The listing builds one solid part. Answer for the finished solid, in the listing's coordinates (mm). A direction names the side the tool comes from. Give positions to 0.01 mm unless a question says otherwise; leave off trailing zeros. One line per question, with ' | ' between items. Start each with the question number.
1. A cutting plane is placed at A-A (z = 21.5). State how many separate pieces and enclosed holes the cut face has, then the cut area to 3 significant figures.
2. Given P1, Ø4.5, axis at x = -23.89, y = 1.91, coming from the +Z side; P2, Ø0.8, axis at x = -17.5, z = 77, coming from the +Y side, each flat-ended and moving along its own axis, determine where each tip first touches the part or whether it passes through.
3. Find the intervals of material crossed by L1, parallel to X at y = 2, z = 43.5; L2, parallel to X at y = 3.75, z = 32; L3, parallel to X at y = 0, z = 39, in increasing order. Write a range as from..to.
4. For faces 1 (the face through (1, 2, 0)), 2 (the face through (-28.891, 4, 60)), determine the directions among +Z, -Z, +X, -X, +Y, -Y from which every point of the face is accessible in a straight line to the end or side of a thin tool.
5. The mould has two halves that part along X. Classify faces 3 (the face through (-18.891, 4, 60)), 4 (the face through (36.109, 2, 60)), 5 (the face through (1, -3.09, 60)): +X half, -X half, draft (parallel to the pull), parting line (faces both ways), or undercut.
```python
from build123d import *

# Parameters (mm, degrees)
ESQUISSE1_R        = 2.8
BOSS_EXTRU_1_DEPTH = 122
CONG_1_R           = 1
CONG_2_R           = 2


with BuildPart() as part:
    # Esquisse1 → Boss.-Extru.1 (new body)
    with BuildSketch(Plane.XY):
        Polygon((-35.89112663, -3.089603204), (-35.89112663, 6.910396796), (-31.89112663, 6.910396796), (-31.89112663, 0.910396796), (-28.89112663, 0.910396796), (-28.89112663, 6.910396796), (-18.89112663, 6.910396796), (-18.89112663, 0.910396796), (-15.89112663, 0.910396796), (-15.89112663, 6.910396796), (23.10887337, 6.910396796), (23.10887337, 0.910396796), (26.10887337, 0.910396796), (26.10887337, 6.910396796), (36.10887337, 6.910396796), (36.10887337, -3.089603204), align=None)
        with Locations((-23.89112663, 1.910396796)):
            Circle(ESQUISSE1_R, mode=Mode.SUBTRACT)
        with Locations((31.10887337, 1.910396796)):
            Circle(ESQUISSE1_R, mode=Mode.SUBTRACT)
    extrude(amount=BOSS_EXTRU_1_DEPTH)

    # Congé1
    cong_1_edges = [part.edges().sort_by_distance(p)[0] for p in [
        (-31.89112663, 0.910396796, 61),
        (-31.89112663, 6.910396796, 61),
        (26.10887337, 6.910396796, 61),
        (26.10887337, 0.910396796, 61),
        (23.10887337, 0.910396796, 61),
        (23.10887337, 6.910396796, 61),
        (-15.89112663, 6.910396796, 61),
        (-15.89112663, 0.910396796, 61),
        (-18.89112663, 0.910396796, 61),
        (-18.89112663, 6.910396796, 61),
        (-28.89112663, 6.910396796, 61),
        (-28.89112663, 0.910396796, 61),
    ]]
    fillet(cong_1_edges, radius=CONG_1_R)

    # Congé2
    cong_2_edges = [part.edges().sort_by_distance(p)[0] for p in [
        (-35.89112663, 6.910396796, 61),
        (-35.89112663, -3.089603204, 61),
        (36.10887337, -3.089603204, 61),
        (36.10887337, 6.910396796, 61),
    ]]
    fillet(cong_2_edges, radius=CONG_2_R)


solid = part.part
```
Determined:
1) separate pieces: 1 | enclosed holes: 2 | area: 613 mm2
2) P1: through | P2: y = 0.91
3) L1: -35.89..-31.89, -28.89..-26.69, -21.09..-18.89, -15.89..23.11, 26.11..28.31, 33.91..36.11 | L2: -35.89..-31.89, -28.89..-26, -21.78..-18.89, -15.89..23.11, 26.11..29, 33.22..36.11 | L3: -35.89..-25.94, -21.84..29.06, 33.16..36.11
4) face 1: -Z, +X, -X, +Y, -Y | face 2: +Z, -Z, +Y
5) face 3: undercut | face 4: +X half | face 5: draft
